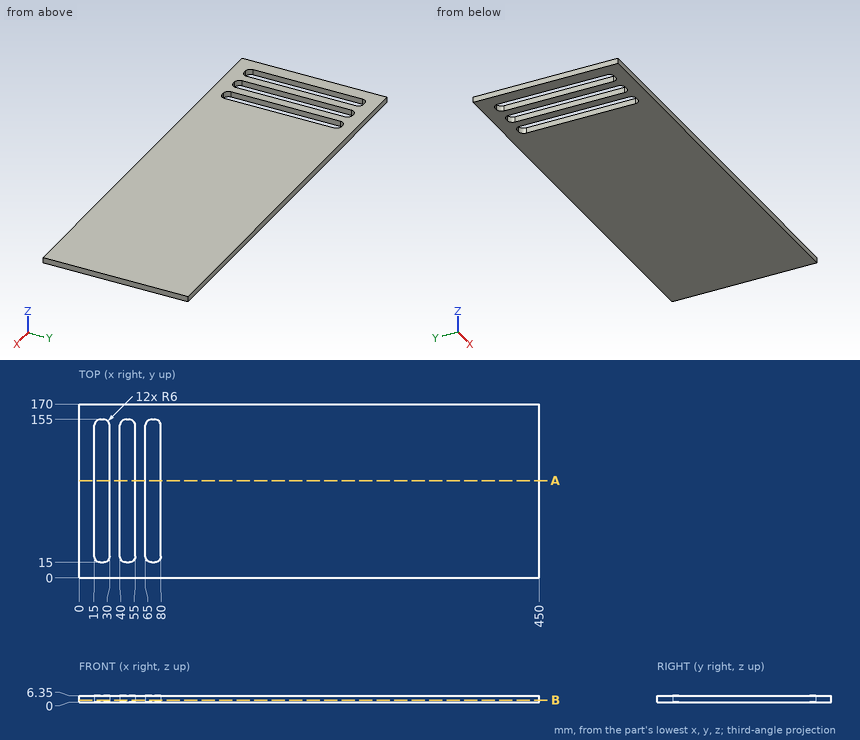
Drawing for the job (mm, zero at the part's lowest x, y, z). Coordinates: 2 decimals unless noted, no trailing zeros. Order: outer loops, then holes, each group sorted by start corner. A loop starts at its lowest first (then second) coordinate and runs counter-clockwise, first axis right, second up. Notation, with made-up numbers: (25, -28.75) -> (58, -28.75) arc R15 cw to (58, -11.75) -> close; hole circle Ø2 at (17, 69). An arc over 180 degrees is marked (long way). Return JSON: item names as keys, results as strings.
Item 1: Wall check: line 1 along X through (y, z) = (37, 3.25); line 2 along Y through (x, z) = (21, 3); line 3 along X through (y, z) = (19.5, 5.75). Give the ranges that are in metal, low to high. Write a range as from..to.
Model answer:
{"line 1": "x = 0..15, 30..40, 55..65, 80..450", "line 2": "y = 0..15, 155..170", "line 3": "x = 0..15.19, 29.81..40.19, 54.81..65.19, 79.81..450"}
Item 2: Slice it at B-B (z = 2.25). Write the cut outline in (x, y), then the cut area to 3 significant figures.
Model answer:
{"outline": "(0, 0) -> (450, 0) -> (450, 170) -> (0, 170) -> close; hole (15, 21) arc R6 ccw to (21, 15) -> (24, 15) arc R6 ccw to (30, 21) -> (30, 149) arc R6 ccw to (24, 155) -> (21, 155) arc R6 ccw to (15, 149) -> close; hole (40, 21) arc R6 ccw to (46, 15) -> (49, 15) arc R6 ccw to (55, 21) -> (55, 149) arc R6 ccw to (49, 155) -> (46, 155) arc R6 ccw to (40, 149) -> close; hole (65, 21) arc R6 ccw to (71, 15) -> (74, 15) arc R6 ccw to (80, 21) -> (80, 149) arc R6 ccw to (74, 155) -> (71, 155) arc R6 ccw to (65, 149) -> close", "area": "70,300 mm²"}
Item 3: Slice it at A-A (y = 95). Write the cut outline in (x, z).
Model answer:
{"outline": "(0, 0) -> (15, 0) -> (15, 6.35) -> (0, 6.35) -> close; (30, 0) -> (40, 0) -> (40, 6.35) -> (30, 6.35) -> close; (55, 0) -> (65, 0) -> (65, 6.35) -> (55, 6.35) -> close; (80, 0) -> (450, 0) -> (450, 6.35) -> (80, 6.35) -> close"}
